Source: CAD feature listing. Evaluate the final solid. Frame: model axes, mm. A direction names the side the tool comes from. Round coordinates to 2 decimals unless told otherwise and drop trailing zeros. Loops run counter-clockwise (first coordinate to the right, second up) from the corner with the lowest first, then second, coordinate; pieces in that order, holes last. Notation, with made-up numbers: (14.25, 25.25) -> (41.25, 25.25) arc R28 ccw to (41.25, 44.25) -> close; hole circle Ø2 at (10.25, 62). An arc over 180 degrees is marked (long way). Put each result on its own line as item: value. Start each with the question number.
1. Cut plane C-C (y = -6). Return the cut outline in (x, z).
2. Cut plane D-D (x = -6). Return the cut outline in (y, z).
3. Material intervals for L1, parallel to X at y = 3, z = -3.25; L2, parallel to Y at x = -2, z = -3.5; L3, parallel to X at y = 6.5, z = 0.75, sorted ascending.
4. Draft query along X for faces 5 (the cylindrical face through (-13.887, -10.648, 0.056)), 6 (the flat face through (0, 10, 2.5)), 7 (the flat face through (-1.2, -1, -5.5)). Return one class per face: pulls with the +X half, pulls with the -X half, needs draft (parallel to the pull), parting line crosses it, or undercut.
5. Cut plane A-A (z = -3). State how many separate pieces and enclosed holes the cut face has, then the cut area to 3 significant figures.
6. Set-up query: faces 1 (the flat face through (-1.2, -1, 5.5)), 2 (the flat face through (8, -5, -2.5)), 3 (the flat face through (6.92, -5.63, 0.04)), 4 (the flat face through (-8, -5, 2.5)). Return all of +Z, -Z, +X, -X, +Y, -Y with unobstructed straight access to the full face (end or side cutting, diameter ignored); none if empty.
7. Contact query for flat-ended pins moving along their axis: pin 1 (4 mm diameter, centred on x = 6.5, y = 11, fed in from +Z); pin 2 (6 mm diameter, centred on x = 4, z = 3, fed in from -Y); pin 3 (5 mm diameter, centred on x = 0, y = 8.5, fed in from +Z). Output: stop coordinate, or through.
```python
from build123d import *

# Parameters (mm, degrees)
F1_DEPTH = 5.5
F2_DEPTH = 2.5
F0_R     = 17.5
F3_DEPTH = 4


with BuildPart() as f1:
    # F0 (on Top) → F1 (new body, symmetric)
    with BuildSketch(Plane.XY):
        with BuildLine():
            ThreePointArc((-1.1691342951, -0.675), (-1.1691342951, 0.675), (0, 1.35))
            Line((0, 1.35), (-0.6846800298, 4.9528994798))
            ThreePointArc((-0.6846800298, 4.9528994798), (-4.3301270189, 2.5), (-4.6316767868, -1.8834994406))
            Line((-4.6316767868, -1.8834994406), (-1.1691342951, -0.675))
        make_face()
        with BuildLine():
            Line((-3.946996757, -3.0694000392), (-1.1691342951, -0.675))
            Line((-1.1691342951, -0.675), (-4.6316767868, -1.8834994406))
            ThreePointArc((-4.6316767868, -1.8834994406), (-4.3301270189, -2.5), (-3.946996757, -3.0694000392))
        make_face()
        with BuildLine():
            ThreePointArc((-3.946996757, -3.0694000392), (0, -5), (3.946996757, -3.0694000392))
            Line((3.946996757, -3.0694000392), (1.1691342951, -0.675))
            ThreePointArc((1.1691342951, -0.675), (0, -1.35), (-1.1691342951, -0.675))
            Line((-1.1691342951, -0.675), (-3.946996757, -3.0694000392))
        make_face()
        with BuildLine():
            ThreePointArc((5, 0), (3.7698408553, 3.284554753), (0.6846800298, 4.9528994798))
            Line((0.6846800298, 4.9528994798), (0, 1.35))
            ThreePointArc((0, 1.35), (0.9545941546, 0.9545941546), (1.35, 0))
            ThreePointArc((1.35, 0), (1.3039998655, -0.3494057109), (1.1691342951, -0.675))
            Line((1.1691342951, -0.675), (4.6316767868, -1.8834994406))
            ThreePointArc((4.6316767868, -1.8834994406), (4.9070553254, -0.9595874286), (5, 0))
        make_face()
        with BuildLine():
            ThreePointArc((3.946996757, -3.0694000392), (4.3301270189, -2.5), (4.6316767868, -1.8834994406))
            Line((4.6316767868, -1.8834994406), (1.1691342951, -0.675))
            Line((1.1691342951, -0.675), (3.946996757, -3.0694000392))
        make_face()
        with BuildLine():
            Line((0, 1.35), (0.6846800298, 4.9528994798))
            ThreePointArc((0.6846800298, 4.9528994798), (0.3431490938, 4.9882109718), (0, 5))
            Line((0, 5), (0, 1.35))
        make_face()
        with BuildLine():
            Line((0, 1.35), (0, 5))
            ThreePointArc((0, 5), (-0.3431490938, 4.9882109718), (-0.6846800298, 4.9528994798))
            Line((-0.6846800298, 4.9528994798), (0, 1.35))
        make_face()
    extrude(amount=F1_DEPTH, both=True)

    # F0 (on Top) → F2 (join, symmetric)
    with BuildSketch(Plane.XY):
        with BuildLine():
            Line((0.6846800298, 4.9528994798), (2.1712380216, 12.775413329))
            ThreePointArc((2.1712380216, 12.775413329), (1.089476247, 12.9127263497), (0, 12.9586056455))
            Line((0, 12.9586056455), (0, 5))
            ThreePointArc((0, 5), (0.3431490938, 4.9882109718), (0.6846800298, 4.9528994798))
        make_face()
        with BuildLine():
            Line((0, 5), (0, 12.9586056455))
            ThreePointArc((0, 12.9586056455), (-1.089476247, 12.9127263497), (-2.1712380216, 12.775413329))
            Line((-2.1712380216, 12.775413329), (-0.6846800298, 4.9528994798))
            ThreePointArc((-0.6846800298, 4.9528994798), (-0.3431490938, 4.9882109718), (0, 5))
        make_face()
        with BuildLine():
            ThreePointArc((-12.1494514976, -4.5073593802), (-11.2224816866, -6.4793028227), (-9.978213476, -8.2680539489))
            Line((-9.978213476, -8.2680539489), (-3.946996757, -3.0694000392))
            ThreePointArc((-3.946996757, -3.0694000392), (-4.3301270189, -2.5), (-4.6316767868, -1.8834994406))
            Line((-4.6316767868, -1.8834994406), (-12.1494514976, -4.5073593802))
        make_face()
        with BuildLine():
            ThreePointArc((9.978213476, -8.2680539489), (11.2224816866, -6.4793028227), (12.1494514976, -4.5073593802))
            Line((12.1494514976, -4.5073593802), (4.6316767868, -1.8834994406))
            ThreePointArc((4.6316767868, -1.8834994406), (4.3301270189, -2.5), (3.946996757, -3.0694000392))
            Line((3.946996757, -3.0694000392), (9.978213476, -8.2680539489))
        make_face()
    extrude(amount=F2_DEPTH, both=True)

    # F0 (on Top) → F3 (join, symmetric)
    with BuildSketch(Plane.XY):
        Circle(F0_R)
        with BuildLine():
            ThreePointArc((2.1712380216, 12.775413329), (9.9010524077, 8.3603003233), (12.9586056455, 0))
            ThreePointArc((12.9586056455, 0), (12.7547130709, -2.2897062594), (12.1494514976, -4.5073593802))
            ThreePointArc((12.1494514976, -4.5073593802), (11.2224816866, -6.4793028227), (9.978213476, -8.2680539489))
            ThreePointArc((9.978213476, -8.2680539489), (0, -12.9586056455), (-9.978213476, -8.2680539489))
            ThreePointArc((-9.978213476, -8.2680539489), (-11.2224816866, -6.4793028227), (-12.1494514976, -4.5073593802))
            ThreePointArc((-12.1494514976, -4.5073593802), (-11.2224816866, 6.4793028227), (-2.1712380216, 12.775413329))
            ThreePointArc((-2.1712380216, 12.775413329), (-1.089476247, 12.9127263497), (0, 12.9586056455))
            ThreePointArc((0, 12.9586056455), (1.089476247, 12.9127263497), (2.1712380216, 12.775413329))
        make_face(mode=Mode.SUBTRACT)
    extrude(amount=F3_DEPTH, both=True)


solid = f1.part
```
Solution:
1. outline: (-16.44, -4) -> (-11.49, -4) -> (-11.49, -2.5) -> (-7.35, -2.5) -> (-7.35, 2.5) -> (-11.49, 2.5) -> (-11.49, 4) -> (-16.44, 4) -> close; (7.35, -2.5) -> (11.49, -2.5) -> (11.49, -4) -> (16.44, -4) -> (16.44, 4) -> (11.49, 4) -> (11.49, 2.5) -> (7.35, 2.5) -> close
2. outline: (-16.44, -4) -> (-11.49, -4) -> (-11.49, 4) -> (-16.44, 4) -> close; (-4.84, -2.5) -> (-2.36, -2.5) -> (-2.36, 2.5) -> (-4.84, 2.5) -> close; (11.49, -4) -> (16.44, -4) -> (16.44, 4) -> (11.49, 4) -> close
3. L1: x = -17.24 to -12.61, -4 to 4, 12.61 to 17.24
3. L2: y = -17.39 to -12.8, -4.58 to 4.58, 12.8 to 17.39
3. L3: x = -16.25 to -11.21, -0.98 to 0.98, 11.21 to 16.25
4. face 5: parting line crosses it
4. face 6: undercut
4. face 7: needs draft
5. separate pieces: 2
5. enclosed holes: 2
5. area: 507 mm^2
6. face 1: +Z, +X, -X, +Y, -Y
6. face 2: -Z
6. face 3: +Z, -Z
6. face 4: +Z
7. pin 1: stops at z = 4
7. pin 2: stops at y = -17.47
7. pin 3: stops at z = 2.5
